```python
from build123d import *

# Parameters (mm, degrees)
SKETCH1_W           = 110
SKETCH1_H           = 65
BOSS_EXTRUDE1_DEPTH = 38
SKETCH2_W           = 106
SKETCH2_H           = 61
CUT_EXTRUDE1_DEPTH  = 36
SKETCH3_W           = 2
SKETCH3_H           = 61
BOSS_EXTRUDE2_DEPTH = 5
FILLET4_R           = 0.5


with BuildPart() as part:
    # Sketch1 → Boss-Extrude1 (new body)
    with BuildSketch(Plane(origin=(0, 0, 0), x_dir=(1, 0, 0), z_dir=(0, 1, 0))):
        with Locations((11.911764706, 4.558823529)):
            Rectangle(SKETCH1_W, SKETCH1_H)
    extrude(amount=BOSS_EXTRUDE1_DEPTH)

    # Sketch2 → Cut-Extrude1 (cut)
    with BuildSketch(Plane(origin=(0, 38, 0), x_dir=(1, 0, 0), z_dir=(0, 1, 0))):
        with Locations((11.911764706, 4.558823529)):
            Rectangle(SKETCH2_W, SKETCH2_H)
    extrude(amount=-CUT_EXTRUDE1_DEPTH, mode=Mode.SUBTRACT)

    # Sketch3 → Boss-Extrude2 (add)
    with BuildSketch(Plane(origin=(0, 2, 0), x_dir=(1, 0, 0), z_dir=(0, 1, 0))):
        with Locations((37.911764706, 4.558823529)):
            Rectangle(SKETCH3_W, SKETCH3_H)
    extrude(amount=BOSS_EXTRUDE2_DEPTH)

    # Fillet4
    fillet4_edges = [part.edges().sort_by_distance(p)[0] for p in [
        (66.911764706, 38, -4.558823529),
        (11.911764706, 38, -37.058823529),
        (-41.088235294, 2, -4.558823529),
        (-41.088235294, 20, 25.941176471),
        (51.911764706, 2, -35.058823529),
        (-41.088235294, 20, -35.058823529),
        (64.911764706, 2, -4.558823529),
        (64.911764706, 20, -35.058823529),
        (-2.088235294, 2, 25.941176471),
        (64.911764706, 20, 25.941176471),
        (-41.088235294, 38, -4.558823529),
        (11.911764706, 38, 25.941176471),
        (64.911764706, 38, -4.558823529),
        (11.911764706, 38, -35.058823529),
        (51.911764706, 2, 25.941176471),
        (-2.088235294, 2, -35.058823529),
        (37.911764706, 7, -35.058823529),
        (38.911764706, 4.5, -35.058823529),
        (36.911764706, 2, -4.558823529),
        (36.911764706, 4.5, -35.058823529),
        (36.911764706, 4.5, 25.941176471),
        (38.911764706, 7, -4.558823529),
        (38.911764706, 4.5, 25.941176471),
        (36.911764706, 7, -4.558823529),
        (37.911764706, 7, 25.941176471),
        (38.911764706, 2, -4.558823529),
        (-43.088235294, 38, -4.558823529),
        (66.911764706, 0, -4.558823529),
        (11.911764706, 0, 27.941176471),
        (-43.088235294, 0, -4.558823529),
        (11.911764706, 38, 27.941176471),
        (-43.088235294, 19, -37.058823529),
        (66.911764706, 19, -37.058823529),
        (66.911764706, 19, 27.941176471),
        (-43.088235294, 19, 27.941176471),
    ]]
    fillet(fillet4_edges, radius=FILLET4_R)


solid = part.part
```
Work out the finished part from the listing and answer in its coordinate system (mm). A direction names the side the tool comes from. Round coordinates to 2 decimals unless told otherwise and drop trailing zeros. Loops run counter-clockwise (first coordinate to the right, second up) from the corner with the lowest first, then second, coordinate; pieces in that order, holes last. Notation, with made-up numbers: M -6.75,-25 L 33.25,-25 A24 ccw 33.25,4 Z; hole C 32,23 d7. An arc over 180 degrees is marked long. One line per question, with ' | ' between items.
Q1. Find section A-A, the plane y = 10. Give the vertices of the cut face in (x, z), then the cut area to 3 significant figures.
Conclusion:
outline: M -43.09,-36.56 A0.5 ccw -42.59,-37.06 L 66.41,-37.06 A0.5 ccw 66.91,-36.56 L 66.91,27.44 A0.5 ccw 66.41,27.94 L -42.59,27.94 A0.5 ccw -43.09,27.44 Z; hole M -41.09,-34.56 A0.5 ccw -40.59,-35.06 L 64.41,-35.06 A0.5 ccw 64.91,-34.56 L 64.91,25.44 A0.5 ccw 64.41,25.94 L -40.59,25.94 A0.5 ccw -41.09,25.44 Z | area: 684 mm2
Q2. A tool of negligible diameter and unlimited length cuts with its end or side. For faces 4 (the flat face through (11, 0, -5)), 5 (the flat face through (64.912, 20, -4)), from which of +Z, -Z, +X, -X, +Y, -Y can it reach the whole face along a straight path? Write none if from no direction.
Conclusion:
face 4: +Z, -Z, +X, -X, -Y | face 5: +Y
Q3. Find section B-B, the plane x = 44.5. Give the vertices of the cut face in (y, z), then the cut area to 3 significant figures.
Conclusion:
outline: M 0,-37.06 L 37.5,-37.06 A0.5 ccw 38,-36.56 L 38,-35.56 A0.5 ccw 37.5,-35.06 L 2.5,-35.06 A0.5 cw 2,-34.56 L 2,25.44 A0.5 cw 2.5,25.94 L 37.5,25.94 A0.5 ccw 38,26.44 L 38,27.44 A0.5 ccw 37.5,27.94 L 0.5,27.94 A0.5 ccw 0,27.44 Z | area: 274 mm2
Q4. Find section C-C, the plane z = 2. Give the vertices of the cut face in (x, y).
Conclusion:
outline: M -43.09,0.5 A0.5 ccw -42.59,0 L 66.41,0 A0.5 ccw 66.91,0.5 L 66.91,37.5 A0.5 ccw 66.41,38 L 65.41,38 A0.5 ccw 64.91,37.5 L 64.91,2.5 A0.5 cw 64.41,2 L 39.41,2 A0.5 cw 38.91,2.5 L 38.91,6.5 A0.5 ccw 38.41,7 L 37.41,7 A0.5 ccw 36.91,6.5 L 36.91,2.5 A0.5 cw 36.41,2 L -40.59,2 A0.5 cw -41.09,2.5 L -41.09,37.5 A0.5 ccw -41.59,38 L -42.59,38 A0.5 ccw -43.09,37.5 Z
Q5. Each of these flat-tipped pins is pushed along its axis until it touches: pin 1 Ø0.8 at (x, z) = (38, -14.5) entering from +Y; pin 2 Ø12.5 at (x, z) = (52, -9.5) entering from +Y. Where does it stop, or does it pass through?
Conclusion:
pin 1: stops at y = 7 | pin 2: stops at y = 2
Q6. The mould has two halves that part along Z. Classify faces 1 (the flat face through (52, 2, -5)), 2 (the flat face through (11, 19, 27.941)), 3 (the flat face through (66.912, 19, -4)): +Z half, -Z half, draft (parallel to the pull), parting line (faces both ways), or undercut.
Conclusion:
face 1: undercut | face 2: +Z half | face 3: draft
Q7. Consider line 1 along X through (y, z) = (5, 18); line 2 along Z through (x, y) = (-6, 26); line 3 along X through (y, z) = (19, 8). Determine where each line is inside the solid, lowest interval first. Write a range as from..to.
Conclusion:
line 1: x = -43.09..-41.09, 36.91..38.91, 64.91..66.91 | line 2: z = -37.06..-35.06, 25.94..27.94 | line 3: x = -43.09..-41.09, 64.91..66.91
